CAD build for the part. Positions are in the model's coordinates, mm. Round coordinates to 2 decimals unless told otherwise and drop trailing zeros. Loops run counter-clockwise (first coordinate to the right, second up) from the corner with the lowest first, then second, coordinate; pieces in that order, holes last.
from build123d import *

# Parameters (mm, degrees)
SKETCH1_W           = 115
SKETCH1_H           = 30
BOSS_EXTRUDE1_DEPTH = 4


with BuildPart() as part:
    # Sketch1 → Boss-Extrude1 (new body)
    with BuildSketch(Plane(origin=(0, 0, 0), x_dir=(1, 0, 0), z_dir=(0, 1, 0))):
        Polygon((57.5, -30), (0, -30), (57.5, -60), align=None)
        with Locations((57.5, -15)):
            Rectangle(SKETCH1_W, SKETCH1_H)
        Polygon((57.5, -30), (57.5, -60), (115, -30), align=None)
    extrude(amount=BOSS_EXTRUDE1_DEPTH)


solid = part.part
Item 1: Cut at C-C (x = 43). List the corners of the cut face in (y, z), plus the area to 3 significant figures.
Verdict:
outline: (0, 0) - (4, 0) - (4, 52.43) - (0, 52.43) - close
area: 210 mm2
Item 2: Cut at B-B (z = 39). List the corners of the cut face in (x, y), plus the area to 3 significant figures.
Verdict:
outline: (17.25, 0) - (97.75, 0) - (97.75, 4) - (17.25, 4) - close
area: 322 mm2
Item 3: Cut at A-A (y = 2.3). List the corners of the cut face in (x, z), plus the area to 4 significant figures.
Verdict:
outline: (0, 0) - (115, 0) - (115, 30) - (57.5, 60) - (0, 30) - close
area: 5,175 mm2
Item 4: Flat gauge pins, fed straight in: P1, Ø1.5, axis at x = 54.5, y = 3.5, coming from the +Z side; P2, Ø2, axis at y = 3.5, z = 48, coming from the -X side. Where does each tip first touch, or does it go through?
Verdict:
P1: stops at z = 58.83
P2: stops at x = 32.58
Item 5: Wall check: L1, parallel to Z at x = 109, y = 3.4; L2, parallel to Z at x = 106.5, y = 2.5; L3, parallel to X at y = 3.1, z = 56.5. Give the ranges that are in metal, low to high.
Verdict:
L1: z = 0 to 33.13
L2: z = 0 to 34.43
L3: x = 50.79 to 64.21
